from build123d import *

# Parameters (mm, degrees)
SKETCH1_W           = 209.55
SKETCH1_H           = 128.5875
BOSS_EXTRUDE1_DEPTH = 88.9
FILLET1_R           = 12.7
FILLET2_R           = 12.7
FILLET3_R           = 12.7
FILLET4_R           = 12.7
SHELL1_T            = -2.54


with BuildPart() as part:
    # Sketch1 → Boss-Extrude1 (new body)
    with BuildSketch(Plane(origin=(0, 0, 0), x_dir=(1, 0, 0), z_dir=(0, 1, 0))):
        with Locations((79.577166722, 28.014941846)):
            Rectangle(SKETCH1_W, SKETCH1_H)
    extrude(amount=BOSS_EXTRUDE1_DEPTH)

    # Fillet1
    fillet1_edges = [part.edges().sort_by_distance(p)[0] for p in [
        (184.352166722, 88.9, -28.014941846),
    ]]
    fillet(fillet1_edges, radius=FILLET1_R)

    # Fillet2
    fillet2_edges = [part.edges().sort_by_distance(p)[0] for p in [
        (-25.197833278, 88.9, -28.014941846),
    ]]
    fillet(fillet2_edges, radius=FILLET2_R)

    # Fillet3
    fillet3_edges = [part.edges().sort_by_distance(p)[0] for p in [
        (-25.197833278, 0, -28.014941846),
    ]]
    fillet(fillet3_edges, radius=FILLET3_R)

    # Fillet4
    fillet4_edges = [part.edges().sort_by_distance(p)[0] for p in [
        (184.352166722, 0, -28.014941846),
    ]]
    fillet(fillet4_edges, radius=FILLET4_R)

    # Shell1
    shell1_openings = [part.faces().sort_by_distance(p)[0] for p in [
        (79.577166722, 44.45, -92.308691846),
    ]]
    offset(amount=SHELL1_T, openings=shell1_openings, kind=Kind.INTERSECTION)


solid = part.part
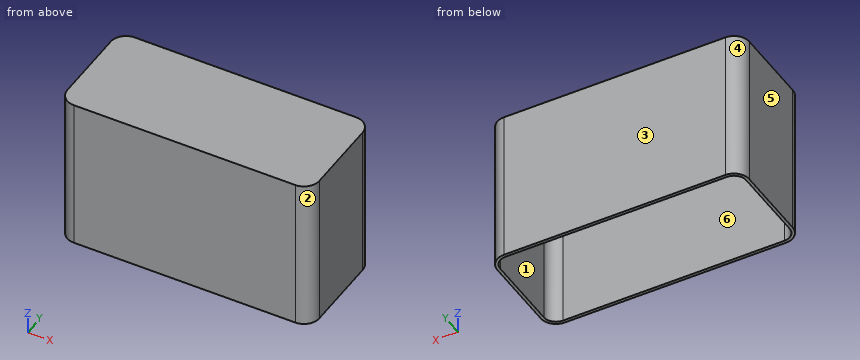
Model file for the job. Use its own axes, mm. Face numbers are marked on the shaded views. A direction names the side the tool comes from. Give positions to 0.01 mm unless a question says otherwise; leave off trailing zeros. Write each loop counter-clockwise with the first axis right and the second up, starting at its lowest first coordinate (ties: lowest second). Pieces come first, ordered by that corner, then holes. Notation, with made-up numbers: M 62.5,63 L 115.5,63 A23 ccw 115.5,85 Z; hole C 4.25,-0.75 d11. An arc over 180 degrees is marked long. One line per item, written item: value. Start each with the question number.
Q1. 3-axis set-ups, long thin cutter, end or side, ignore diameter. For the marked faces 5 and 6: which of +Z, -Z, +X, -X, +Y, -Y reach the whole face in a straight line?
Q2. Saw through at A-A, the plane y = 71.5. Write the cut outline in (x, z).
Q3. Saw through at C-C, the plane x = 97.5. Write the cut outline in (y, z).
Q4. Drop a flat-ended pin along its axis: pin 1 Ø3 at (x, y) = (131, 67) entering from -Z. Give the stop position or say it passes through.
Q5. Two-plate mould, pull along X, no slides. Class the marked faces 1, 2, 3 and 4: +X half, -X half, draft (parallel to the pull), parting line (faces both ways), or undercut.
Q6. Saw through at B-B, the plane z = -53. Write the cut outline in (x, y), plus the area to 3 significant figures.
Q7. Probe probe 1 along X at (y, z) = (58, 10); probe 2 along Y at (x, z) = (50, 29.5); probe 3 along Y at (x, z) = (-13, 21). List the from-to ranges inside material, lowest first. Write a range as [from, to].
Output values:
1. face 5: +Z, -Z, -X, +Y, -Y
1. face 6: -Z
2. outline: M -25.2,-92.31 L -22.66,-92.31 L -22.66,33.74 L 181.81,33.74 L 181.81,-92.31 L 184.35,-92.31 L 184.35,36.28 L -25.2,36.28 Z
3. outline: M 0,-92.31 L 2.54,-92.31 L 2.54,33.74 L 86.36,33.74 L 86.36,-92.31 L 88.9,-92.31 L 88.9,36.28 L 0,36.28 Z
4. pin 1: stops at z = 33.74
5. face 1: undercut
5. face 2: +X half
5. face 3: draft
5. face 4: -X half
6. outline: M -25.2,12.7 A12.7 ccw -12.5,0 L 171.65,0 A12.7 ccw 184.35,12.7 L 184.35,76.2 A12.7 ccw 171.65,88.9 L -12.5,88.9 A12.7 ccw -25.2,76.2 Z; hole M -22.66,12.7 A10.16 ccw -12.5,2.54 L 171.65,2.54 A10.16 ccw 181.81,12.7 L 181.81,76.2 A10.16 ccw 171.65,86.36 L -12.5,86.36 A10.16 ccw -22.66,76.2 Z
6. area: 1,440 mm²
7. probe 1: x = [-25.2, -22.66], [181.81, 184.35]
7. probe 2: y = [0, 2.54], [86.36, 88.9]
7. probe 3: y = [0.01, 2.55], [86.35, 88.89]
